```python
from build123d import *

# Parameters (mm, degrees)
BASE_FLANGE1_DEPTH  = 50.8
MITER_START         = -18.685
MITER_FLANGE2_DEPTH = 37.37
SKETCH24_W          = 6.35
SKETCH24_H          = 12.7
CUT_EXTRUDE1_DEPTH  = 3.175


# Read off the part's stored shape, not the designer's step: Miter Flange2
# Sheet-metal steps are written as plain solids
with BuildPart() as part:
    # Sketch1 → Base-Flange1 (new body)
    with BuildSketch(Plane(origin=(0, 0, 0), x_dir=(1, 0, 0), z_dir=(0, 1, 0))):
        with BuildLine():
            Line((-22.86, 76.2), (-22.86, 4.175))
            ThreePointArc((-22.86, 4.175), (-21.637170811, 1.222829189), (-18.685, 0))
            Line((-18.685, 0), (18.685, 0))
            ThreePointArc((18.685, 0), (21.637170811, 1.222829189), (22.86, 4.175))
            Line((22.86, 4.175), (22.86, 76.2))
            Line((22.86, 76.2), (19.685, 76.2))
            Line((19.685, 76.2), (19.685, 4.175))
            ThreePointArc((19.685, 4.175), (19.392106781, 3.467893219), (18.685, 3.175))
            Line((18.685, 3.175), (-18.685, 3.175))
            ThreePointArc((-18.685, 3.175), (-19.392106781, 3.467893219), (-19.685, 4.175))
            Line((-19.685, 4.175), (-19.685, 76.2))
            Line((-19.685, 76.2), (-22.86, 76.2))
        make_face()
    extrude(amount=BASE_FLANGE1_DEPTH)

    # Miter Flange2 outline → Miter Flange2 (add)
    with BuildSketch(Plane.YZ.offset(MITER_START)):
        with BuildLine():
            Line((-29.600045956, -27.870704333), (-27.354981926, -30.115768363))
            Line((-27.354981926, -30.115768363), (-0.707106781, -3.467893219))
            ThreePointArc((-0.707106781, -3.467893219), (-0.382683432, -3.251120467), (0, -3.175))
            Line((0, -3.175), (0, 0))
            ThreePointArc((0, 0), (-1.59770333, -0.317802952), (-2.952170811, -1.222829189))
            Line((-2.952170811, -1.222829189), (-29.600045956, -27.870704333))
        make_face()
    extrude(amount=MITER_FLANGE2_DEPTH)

    # Sketch24 → Cut-Extrude1 (cut)
    with BuildSketch(Plane.ZY.offset(22.86)):
        with Locations((-73.025, 44.45)):
            Rectangle(SKETCH24_W, SKETCH24_H)
        with Locations((-73.025, 6.35)):
            Rectangle(SKETCH24_W, SKETCH24_H)
    cut_extrude1 = extrude(amount=-CUT_EXTRUDE1_DEPTH, mode=Mode.SUBTRACT)

    # Mirror2: Cut-Extrude1 across plane
    add(cut_extrude1.mirror(Plane.ZY), mode=Mode.SUBTRACT)


solid = part.part
```
Work out the finished part from the listing and answer in its coordinate system (mm). A direction names the side the tool comes from. Round coordinates to 2 decimals unless told otherwise and drop trailing zeros. Loops run counter-clockwise (first coordinate to the right, second up) from the corner with the lowest first, then second, coordinate; pieces in that order, holes last. Notation, with made-up numbers: M -27.75,-28 L -21.75,-28 A10 ccw -21.75,-15 Z; hole C 14.5,56.25 d4. An arc over 180 degrees is marked long. Use CSV: the item, a comma, the result in double quotes.
Q1. Section D-D, the plane z = -25.5 is taken. Determine the outline of the cut face in (x, y) (3 decimals).
Determined:
outline,"M -22.86,0 L -19.685,0 L -19.685,50.8 L -22.86,50.8 Z; M -18.685,-27.229 L 18.685,-27.229 L 18.685,-22.739 L -18.685,-22.739 Z; M 19.685,0 L 22.86,0 L 22.86,50.8 L 19.685,50.8 Z"
Q2. The mould has two halves that part along X. Classify faces 4 (the cylindrical face through (21.605, 25.044, -1.191)), 5 (the flat face through (0, 25, -3.175)), 6 (the flat face through (-20, 50.8, -30)): pulls with the +X half, pulls with the -X half, needs draft (parallel to the pull), parting line crosses it, or undercut.
Determined:
face 4,"pulls with the +X half"
face 5,"undercut"
face 6,"needs draft"
Q3. Section C-C, the plane y = 23 is taken. Determine the outline of the cut face in (x, z) (3 decimals), then the cut area to 3 significant figures.
Determined:
outline,"M -22.86,-76.2 L -19.685,-76.2 L -19.685,-4.175 A1 cw -18.685,-3.175 L 18.685,-3.175 A1 cw 19.685,-4.175 L 19.685,-76.2 L 22.86,-76.2 L 22.86,-4.175 A4.175 ccw 18.685,0 L -18.685,0 A4.175 ccw -22.86,-4.175 Z"
area,"602 mm2"
Q4. A tool of negligible diameter and unlimited length cuts with its end or side. For faces 1 (the flat face through (-19.685, 25, -40)), 2 (the flat face through (-21, 44, -69.85)), 3 (the flat face through (-21, 12.7, -73)), from which of +Z, -Z, +X, -X, +Y, -Y can it reach the whole face along a straight path? Write none if from no direction.
Determined:
face 1,"-Z, +Y, -Y"
face 2,"-Z, +X, -X, +Y"
face 3,"-Z, +X, -X, -Y"
Q5. Each of these flat-tipped pins is pushed along its axis until it touches: pin 1 (10 mm diameter, centred on x = -5, z = -29.5, fed in from +Y); pin 2 (2.5 mm diameter, centred on x = 22, z = -72.5, fed in from -Y); pin 3 (2.5 mm diameter, centred on x = -21, y = 8, fed in from -Z); pin 4 (12 mm diameter, centred on x = 15, z = -56.5, fed in from +Y). Where does it stop, or does it pass through?
Determined:
pin 1,"y = -21.74"
pin 2,"y = 12.7"
pin 3,"z = -69.85"
pin 4,"y = 50.8"
Q6. Section B-B, the plane x = -10 is taken. Determine the outline of the cut face in (y, z) (3 decimals), then the cut area to 3 significant figures.
Determined:
outline,"M -29.6,-27.871 L -27.355,-30.116 L -0.707,-3.468 A1 cw 0,-3.175 L 50.8,-3.175 L 50.8,0 L 0,0 A4.175 ccw -2.952,-1.223 Z"
area,"287 mm2"
Q7. Consider L1, parallel to X at y = 43.5, z = -58 (3 decimals); L2, parallel to Z at x = -18, y = 31 (3 decimals); L3, parallel to Y at x = -20, z = -45.5. Determine where each line is inside the solid, lowest interval first.
Determined:
L1,"-22.86 to -19.685, 19.685 to 22.86"
L2,"-3.175 to 0"
L3,"0 to 50.8"
Q8. Section A-A, the plane z = -44.5 is taken. Determine the outline of the cut face in (x, y) (3 decimals).
Determined:
outline,"M -22.86,0 L -19.685,0 L -19.685,50.8 L -22.86,50.8 Z; M 19.685,0 L 22.86,0 L 22.86,50.8 L 19.685,50.8 Z"
